The model under review builds one solid part; all positions refer to its coordinate system, in mm. Face numbers are marked on the shaded views. Round coordinates to 2 decimals unless told otherwise and drop trailing zeros. Order: outer loops, then holes, each group sorted by start corner. A loop starts at its lowest first (then second) coordinate and runs counter-clockwise, first axis right, second up. Notation, with made-up numbers: (-9, -33) -> (20, -33) arc R30 ccw to (20, 0) -> close; hole circle Ø2 at (-20.75, -8.5). An arc over 180 degrees is marked (long way). Put each result on its own line as item: value. Start each with the question number.
Autodesk Inventor part; units mm, degrees
ref_plane "YZ Plane" through (0, 0, 0) normal (1, 0, 0) x (0, 1, 0)
ref_plane "XZ Plane" through (0, 0, 0) normal (0, 1, 0) x (-1, 0, 0)
ref_plane "XY Plane" through (0, 0, 0) normal (0, 0, 1) x (1, 0, 0)
sketch "Sketch1" plane through (0, 0, 0) normal (0, 0, 1) x (1, 0, 0)
  line L0 (0, 0) -> (101.6, 0)
  line L1 (101.6, 0) -> (101.6, 50.8)
  line L2 (101.6, 50.8) -> (0, 50.8)
  line L3 (0, 50.8) -> (0, 0)
  dimension "d0" = 101.6
  dimension "d1" = 50.8
extrude "Extrusion1" add sketch "Sketch1" along normal blind 6.35
fillet "Fillet1" radius 7.62 4 edges at (101.6, 50.8, 3.175) (101.6, 0, 3.175) (0, 50.8, 3.175) (0, 0, 3.175)
sketch "Sketch2" plane through (0, 0, 6.35) normal (0, 0, 1) x (1, 0, 0)
  circle A0 centre (25.4, 25.4) radius 20.8748
  line L0 (101.6, 7.62) -> (101.6, 43.18)
  circle A1 centre (25.4, 25.4) radius 17.78
  point P0 (0, 0)
  dimension "d5" = 76.2
  dimension "d13" = 3.0948
extrude "Extrusion2" add sketch "Sketch2" along normal blind 6.35 contours A0 | A1
extrude "Extrusion3" cut sketch "Sketch2" along normal blind 6.35 contours A1
extrude "Extrusion4" add sketch "Sketch2" along normal blind 3.81 contours A1
fillet "Fillet3" radius 1.5474 2 edges at (4.5252, 25.4, 12.7) (7.62, 25.4, 12.7)
sketch "Sketch3" plane through (0, 0, 6.35) normal (0, 0, 1) x (1, 0, 0)
  line L0 (60.7255, 39.2684) -> (73.4255, 39.2684)
  line L1 (73.4255, 39.2684) -> (73.4255, 26.5684)
  line L2 (73.4255, 26.5684) -> (60.7255, 26.5684)
  line L3 (60.7255, 26.5684) -> (60.7255, 39.2684)
  line L4 (60.7255, 11.5316) -> (73.4255, 11.5316)
  line L5 (73.4255, 11.5316) -> (73.4255, 24.2316)
  line L6 (73.4255, 24.2316) -> (60.7255, 24.2316)
  line L7 (60.7255, 24.2316) -> (60.7255, 11.5316)
  line L8 (93.98, 50.8) -> (7.62, 50.8)
  line L9 (7.62, 0) -> (93.98, 0)
  point P0 (0, 0)
  dimension "d15" = 12.7
  dimension "d16" = 12.7
  dimension "d17" = 12.7
  dimension "d18" = 12.7
  dimension "d19" = 11.5316
  dimension "d20" = 11.5316
extrude "Extrusion5" add sketch "Sketch3" along normal blind 3.81
chamfer "Chamfer1" distance 1.5875 angle 45 4 edges at (67.0755, 39.2684, 10.16) (73.4255, 32.9184, 10.16) (67.0755, 26.5684, 10.16) (60.7255, 32.9184, 10.16)
chamfer "Chamfer2" distance 1.5875 angle 45 4 edges at (67.0755, 24.2316, 10.16) (60.7255, 17.8816, 10.16) (67.0755, 11.5316, 10.16) (73.4255, 17.8816, 10.16)
sketch "Sketch4" plane through (0, 0, 10.16) normal (0, 0, 1) x (1, 0, 0)
  line L0 (64.1926, 30.4165) -> (67.0755, 35.4098)
  line L1 (64.1926, 30.4165) -> (69.9584, 30.4165) construction
  line L2 (67.0755, 35.4098) -> (69.9584, 30.4165)
  line L3 (69.9584, 30.4165) -> (64.1926, 30.4165)
  line L4 (62.313, 28.1559) -> (62.313, 37.6809)
  line L5 (71.838, 37.6809) -> (71.838, 28.1559)
  line L6 (71.838, 28.1559) -> (62.313, 28.1559)
  line L7 (64.1926, 20.3835) -> (69.9584, 20.3835)
  line L8 (69.9584, 20.3835) -> (67.0755, 15.3902)
  line L9 (67.0755, 15.3902) -> (64.1926, 20.3835)
  line L10 (62.313, 22.6441) -> (71.838, 22.6441)
  line L11 (62.313, 13.1191) -> (62.313, 22.6441)
  point P0 (0, 0)
  dimension "d29" = 60
  dimension "d30" = 60
  dimension "d31" = 1.8796
  dimension "d33" = 5.7658
  dimension "d35" = 2.2606
  dimension "d36" = 4.9933
  dimension "d37" = 5.7658
  dimension "d38" = 5.7658
  dimension "d39" = 60
  dimension "d40" = 2.2606
  dimension "d41" = 1.8796
extrude "Extrusion6" cut sketch "Sketch4" against normal blind 0.381
sketch "Sketch5" plane through (0, 0, 6.35) normal (0, 0, 1) x (1, 0, 0)
  line L0 (81.1657, 31.75) -> (93.8657, 31.75)
  line L1 (93.8657, 31.75) -> (93.8657, 19.05)
  line L2 (93.8657, 19.05) -> (81.1657, 19.05)
  line L3 (81.1657, 19.05) -> (81.1657, 31.75)
  line L4 (93.98, 50.8) -> (7.62, 50.8)
  line L5 (101.6, 7.62) -> (101.6, 43.18)
  point P0 (0, 0)
  dimension "d44" = 12.7
  dimension "d45" = 12.7
  dimension "d46" = 19.05
  dimension "d47" = 7.7343
extrude "Extrusion7" add sketch "Sketch5" along normal blind 3.81
chamfer "Chamfer3" distance 1.5875 angle 45 4 edges at (87.5157, 31.75, 10.16) (93.8657, 25.4, 10.16) (87.5157, 19.05, 10.16) (81.1657, 25.4, 10.16)
fillet "Fillet4" radius 1.0316 8 edges at (2.2318, 48.5682, 6.35) (0, 25.4, 6.35) (2.2318, 2.2318, 6.35) (50.8, 0, 6.35) (99.3682, 2.2318, 6.35) (101.6, 25.4, 6.35) (99.3682, 48.5682, 6.35) (50.8, 50.8, 6.35)
fillet "Fillet5" radius 1.0316 8 edges at (2.2318, 48.5682, 0) (0, 25.4, 0) (2.2318, 2.2318, 0) (50.8, 0, 0) (99.3682, 2.2318, 0) (101.6, 25.4, 0) (99.3682, 48.5682, 0) (50.8, 50.8, 0)
properties part number "Control Panel"
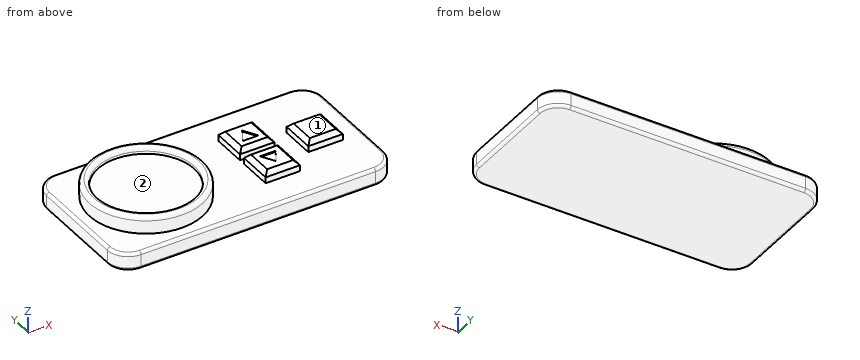
Q1. Take a section at C-C on x = 50. Give the boundary of the cut face in (y, z), and give its area (3 significant figures).
Q2. Draft analysis for pull direction Y (two halves, no side actions). For the marked faces 1 and 2, state which applies: +Y half, -Y half, draft (parallel to the pull), parting line (faces both ways), or undercut.
Q3. Wall thickness on probe 1 along Y at (x, z) = (25.4, 10.5); probe 2 along Z at (x, y) = (42.5, 7.5); probe 3 along Z at (x, y) = (64, 22): over which ranges is each line inside the solid? List them lowest first. Write a range as [from, to].
Q4. Clearance check with flat-ended pins moving along their axes: pin 1 Ø1.8 at (y, z) = (19.5, 7.5) entering from -X; pin 2 Ø8 at (x, y) = (13.5, 26.5) entering from +Z; pin 3 Ø14.5 at (x, y) = (54, 25) entering from +Z; pin 4 Ø1.5 at (x, z) = (53.5, 3) entering from -Y. State where each tip first meets the part, or that it passes through.
Q5. Take a section at D-D on x = 91. Give the boundary of the cut face in (y, z).
Calculated:
1. outline: (0, 1.03) arc R1.03 ccw to (1.03, 0) -> (49.77, 0) arc R1.03 ccw to (50.8, 1.03) -> (50.8, 5.32) arc R1.03 ccw to (49.77, 6.35) -> (1.03, 6.35) arc R1.03 ccw to (0, 5.32) -> close
1. area: 322 mm²
2. face 1: draft
2. face 2: undercut
3. probe 1: y = [4.53, 7.62], [43.18, 46.27]
3. probe 2: z = [0, 6.35]
3. probe 3: z = [0, 10.16]
4. pin 1: stops at x = 5.13
4. pin 2: stops at z = 10.16
4. pin 3: stops at z = 9
4. pin 4: stops at y = 0
5. outline: (0, 1.03) arc R1.03 ccw to (1.03, 0) -> (49.77, 0) arc R1.03 ccw to (50.8, 1.03) -> (50.8, 5.32) arc R1.03 ccw to (49.77, 6.35) -> (31.75, 6.35) -> (31.75, 8.57) -> (30.16, 10.16) -> (20.64, 10.16) -> (19.05, 8.57) -> (19.05, 6.35) -> (1.03, 6.35) arc R1.03 ccw to (0, 5.32) -> close
